from build123d import *

# Parameters (mm, degrees)
F1_DEPTH    = 5.5
F2_DEPTH    = 6.5
F3_T2_ANGLE = 180
F3_T4_ANGLE = 180
F4_R        = 2.5
F5_DEPTH    = 25.4


# Not quite as in the source:
# - a fillet or chamfer that OpenCascade refuses, or shapes differently, is made with other operations: its cross-section is extruded or revolved along the edge and cut away or added


with BuildPart() as f1:
    # F0 (on Front) → F1 (new body, symmetric)
    with BuildSketch(Plane.XZ):
        with BuildLine():
            ThreePointArc((19, 0), (0, -19), (-19, 0))
            Line((-19, 0), (-21, 0))
            ThreePointArc((-21, 0), (0, -21), (21, 0))
            Line((21, 0), (19, 0))
        make_face()
        with BuildLine():
            ThreePointArc((21, 0), (0, -21), (-21, 0))
            Line((-21, 0), (-30, 0))
            Line((-30, 0), (-30, -18.0277563773))
            Line((-30, -18.0277563773), (-18.7349939952, -18.0277563773))
            ThreePointArc((-18.7349939952, -18.0277563773), (0, -26), (18.7349939952, -18.0277563773))
            Line((18.7349939952, -18.0277563773), (30, -18.0277563773))
            Line((30, -18.0277563773), (30, 0))
            Line((30, 0), (21, 0))
        make_face()
    extrude(amount=F1_DEPTH, both=True)

    # F0 (on Front) → F2 (join, symmetric)
    with BuildSketch(Plane.XZ):
        with BuildLine():
            ThreePointArc((19, 0), (0, -19), (-19, 0))
            Line((-19, 0), (-21, 0))
            ThreePointArc((-21, 0), (0, -21), (21, 0))
            Line((21, 0), (19, 0))
        make_face()
    extrude(amount=F2_DEPTH, both=True)

    # F3: fillet of radius 2 on 2 edges, made by hand

    # F3_s1 → F3_t2 (revolve)
    with BuildSketch(Plane.XY):
        with BuildLine():
            ThreePointArc((-22.7320508076, 5.5), (-21.7320508076, 5.7679491924), (-21, 6.5))
            Line((-21, 6.5), (-21, 5.5))
            Line((-21, 5.5), (-22.7320508076, 5.5))
        make_face()
    revolve(axis=Axis((0, 5.5, 0), (0, -1, 0)), revolution_arc=F3_T2_ANGLE)

    # F3_s3 → F3_t4 (revolve)
    with BuildSketch(Plane.XY):
        with BuildLine():
            ThreePointArc((-21, -6.5), (-21.7320508076, -5.7679491924), (-22.7320508076, -5.5))
            Line((-22.7320508076, -5.5), (-21, -5.5))
            Line((-21, -5.5), (-21, -6.5))
        make_face()
    revolve(axis=Axis((0, -5.5, 0), (0, -1, 0)), revolution_arc=F3_T4_ANGLE)

    # F4 (on Top) → F5 (cut)
    with BuildSketch(Plane.XY):
        with Locations((-26, 0)):
            Circle(F4_R)
        with Locations((26, 0)):
            Circle(F4_R)
    extrude(amount=-F5_DEPTH, mode=Mode.SUBTRACT)


solid = f1.part
For this review, take the finished solid that the model builds, in its own axes (mm). A direction names the side the tool comes from. Round coordinates to 2 decimals unless told otherwise and drop trailing zeros. Order: outer loops, then holes, each group sorted by start corner. A loop starts at its lowest first (then second) coordinate and runs counter-clockwise, first axis right, second up. Notation, with made-up numbers: M 15,-7.75 L 73,-7.75 A12 cw 73,13.25 Z; hole C -34,59.25 d6. An arc over 180 degrees is marked long. Use a Markdown table: item, result. Add a question column.
Item 1: Mouldability with a two-part tool opening along Y and no side actions: class faces 6 (the flat face through (0, -6.5, -20)), 7 (the cylindrical face through (23.5, 0.1, -8.9)), 8 (the flat face through (-30, 0, -9)) as released by +Y, released by -Y, zero draft, split by the parting line, or undercut.
Item 2: Add section D-D, the plane z = -14.75. State how many separate pieces and enclosed holes the cut face has, then the cut area to 3 significant figures.
Item 3: Add section A-A, the plane x = 26. Give the boundary of the cut face in (y, z), then the cut area to 3 significant figures.
Item 4: Tool access review of faces 1 (the flat face through (-5, 5.5, -23)), 2 (the flat face through (-23, 0, -18.028)), 3 (the flat face through (-5, -5.5, -23)), 4 (the flat face through (23, 0, -18.028)), 5 (the flat face through (-23, 0, 0)): name each direction out of +Z, -Z, +X, -X, +Y, -Y from which nothing blocks a thin tool from reaching the whole face with its end or side.
Item 5: Add section B-B, the plane y = 0. Give the boundary of the cut face in (x, z) (3 decimals), then the cut area to 3 significant figures.
Item 6: Add section C-C, the plane x = 0. Give the boundary of the cut face in (y, z), then the cut area to 3 significant figures.
Item 7: To check wall thickness, follow line 1 along Y through (x, z) = (-26, -9); line 2 along X through (y, z) = (2.25, -16); line 3 along Y through (x, z) = (-20, -11.25). State the ranges of each line that lie inside material, in increasing order.
Item 8: Insertion check: pin 1 (6 mm diameter, centred on x = 8.5, y = -3.5, fed in from -Z); pin 2 (4 mm diameter, centred on x = 4.5, y = -5, fed in from +Z); pin 3 (1.5 mm diameter, centred on x = -2, y = -4, fed in from -Z). Each pin has a flat end and moves straight along its axis. Give the tip position at first contact, or say it passes through.
Geometry results:
| question | item | result |
|---|---|---|
| 1 | face 6 | released by -Y |
| 1 | face 7 | undercut |
| 1 | face 8 | zero draft |
| 2 | separate pieces | 2 |
| 2 | enclosed holes | 2 |
| 2 | area | 372 mm² |
| 3 | outline | M -5.5,-18.03 L -2.5,-18.03 L -2.5,0 L -5.5,0 Z; M 2.5,-18.03 L 5.5,-18.03 L 5.5,0 L 2.5,0 Z |
| 3 | area | 108 mm² |
| 4 | face 1 | -Z, +Y |
| 4 | face 2 | -Z, -X, +Y, -Y |
| 4 | face 3 | -Z, -Y |
| 4 | face 4 | -Z, +X, +Y, -Y |
| 4 | face 5 | +Z, +X, -X, +Y, -Y |
| 5 | outline | M -30,-18.028 L -28.5,-18.028 L -28.5,0 L -30,0 Z; M -23.5,-18.028 L -18.735,-18.028 A26 ccw 18.735,-18.028 L 23.5,-18.028 L 23.5,0 L 19,0 A19 cw -19,0 L -23.5,0 Z; M 28.5,-18.028 L 30,-18.028 L 30,0 L 28.5,0 Z |
| 5 | area | 541 mm² |
| 6 | outline | M -6.5,-21 A2 cw -5.5,-22.73 L -5.5,-26 L 5.5,-26 L 5.5,-22.73 A2 cw 6.5,-21 L 6.5,-19 L -6.5,-19 Z |
| 6 | area | 82.0 mm² |
| 7 | line 1 | y = -5.5 to -2.5, 2.5 to 5.5 |
| 7 | line 2 | x = -30 to -27.09, -24.91 to -10.25, 10.25 to 24.91, 27.09 to 30 |
| 7 | line 3 | y = -5.5 to 5.5 |
| 8 | pin 1 | stops at z = -25.41 |
| 8 | pin 2 | stops at z = -17.85 |
| 8 | pin 3 | stops at z = -25.97 |
